```python
from build123d import *

# Parameters (mm, degrees)
SKETCH1_R           = 5
BOSS_EXTRUDE1_DEPTH = 15
SKETCH3_W           = 30
SKETCH3_H           = 60
CUT_EXTRUDE2_DEPTH  = 8.5


with BuildPart() as part:
    # Sketch1 → Boss-Extrude1 (new, symmetric)
    with BuildSketch(Plane(origin=(0, 0, 0), x_dir=(0, 0, -1), z_dir=(1, 0, 0))):
        with BuildLine():
            Line((-10, 30), (10, 30))
            Line((10, 30), (36.455619112, 7.637079408))
            ThreePointArc((36.455619112, 7.637079408), (40, 0), (36.455619112, -7.637079408))
            Line((36.455619112, -7.637079408), (10, -30))
            Line((10, -30), (-10, -30))
            Line((-10, -30), (-36.455619112, -7.637079408))
            ThreePointArc((-36.455619112, -7.637079408), (-40, 0), (-36.455619112, 7.637079408))
            Line((-36.455619112, 7.637079408), (-10, 30))
        make_face()
        with Locations((-30, 0)):
            Circle(SKETCH1_R, mode=Mode.SUBTRACT)
        with Locations(Location((30, 0, 0), (0, 0, 180))):
            Circle(SKETCH1_R, mode=Mode.SUBTRACT)
    extrude(amount=BOSS_EXTRUDE1_DEPTH, both=True)

    # Sketch3 → Cut-Extrude2 (cut, symmetric)
    with BuildSketch(Plane(origin=(0, 0, 0), x_dir=(0, 0, -1), z_dir=(1, 0, 0))):
        with Locations((-25, 0)):
            Rectangle(SKETCH3_W, SKETCH3_H)
        with Locations((25, 0)):
            Rectangle(SKETCH3_W, SKETCH3_H)
    extrude(amount=CUT_EXTRUDE2_DEPTH, both=True, mode=Mode.SUBTRACT)


solid = part.part
```
CAD build for the part. Positions are in the model's coordinates, mm. A direction names the side the tool comes from. Coordinates: 2 decimals unless noted, no trailing zeros. Order: outer loops, then holes, each group sorted by start corner. A loop starts at its lowest first (then second) coordinate and runs counter-clockwise, first axis right, second up. Notation, with made-up numbers: M 64.5,-30.75 L 93.5,-30.75 A21 ccw 93.5,-21.75 Z; hole C -39.75,78 d11. An arc over 180 degrees is marked long. Write each question's results on one line, items separated by ' | '. Start each with the question number.
Q1. Drill centre lines: probe 1 along X at (y, z) = (-8, 13); probe 2 along Y at (x, z) = (12.5, 30); probe 3 along Z at (x, y) = (-4.5, 16). Where is each one in solid material? Low to high. Write a range as from..to.
Q2. Cut at A-A (x = -11.5). List the corners of the cut face in (y, z), then the cut area to 3 significant figures.
Q3. Cut at B-B (y = 0). List the corners of the cut face in (x, z).
Q4. Flat gauge pins, fed straight in: P1, Ø12, axis at x = 3.5, z = 27.5, coming from the +Y side; P2, Ø8, axis at x = 10, y = 17, coming from the +Z side; P3, Ø2, axis at x = -9.5, z = -29.5, coming from the +Y side. Where does each tip first touch, or does it go through?
Q5. Cut at C-C (z = -11.5). List the corners of the cut face in (x, y), then the cut area to 3 significant figures.
Q6. Cut at D-D (z = 30). List the corners of the cut face in (x, y), then the cut area to 3 significant figures.
Q7. Which spindle directions (+Z, -Z, +X, -X, +Y, -Y) get a long thin tool onto all of the face, cutting with end or side? Do faces 5 (the flat face through (0, 0, 10)), 6 (the flat face through (0, 0, -10)), 7 (the cylindrical face through (-12, 0, -40)). Say none if no direction does.
Q8. Pull direction Y, two halves, no side cores. Call faces 1 (the cylindrical face through (-12, 0, -35)), 2 (the flat face through (-11.704, 18.662, 23.413)), 3 (the cylindrical face through (12, 0, 35)), 4 (the flat face through (-8.5, 0, -21)): +Y half, -Y half, draft (parallel to the pull), parting line (faces both ways), or undercut.
Found:
1) probe 1: -15..-8.5, 8.5..15 | probe 2: -13.09..-5, 5..13.09 | probe 3: -10..10
2) outline: M -30,-10 L -7.64,-36.46 A10 ccw 7.64,-36.46 L 30,-10 L 30,10 L 7.64,36.46 A10 ccw -7.64,36.46 L -30,10 Z; hole C 0,-30 d10; hole C 0,30 d10 | area: 3,110 mm²
3) outline: M -15,-40 L -8.5,-40 L -8.5,-35 L -15,-35 Z; M -15,-25 L -8.5,-25 L -8.5,-10 L 8.5,-10 L 8.5,-25 L 15,-25 L 15,25 L 8.5,25 L 8.5,10 L -8.5,10 L -8.5,25 L -15,25 Z; M -15,35 L -8.5,35 L -8.5,40 L -15,40 Z; M 8.5,-40 L 15,-40 L 15,-35 L 8.5,-35 Z; M 8.5,35 L 15,35 L 15,40 L 8.5,40 Z
4) P1: y = 18.01 | P2: z = 30.11 | P3: y = 14.36
5) outline: M -15,-28.73 L -8.5,-28.73 L -8.5,28.73 L -15,28.73 Z; M 8.5,-28.73 L 15,-28.73 L 15,28.73 L 8.5,28.73 Z | area: 747 mm²
6) outline: M -15,-13.09 L -8.5,-13.09 L -8.5,-5 L -15,-5 Z; M -15,5 L -8.5,5 L -8.5,13.09 L -15,13.09 Z; M 8.5,-13.09 L 15,-13.09 L 15,-5 L 8.5,-5 Z; M 8.5,5 L 15,5 L 15,13.09 L 8.5,13.09 Z | area: 210 mm²
7) face 5: +Z, +Y, -Y | face 6: -Z, +Y, -Y | face 7: -Z, +X, -X
8) face 1: undercut | face 2: +Y half | face 3: undercut | face 4: draft
